Here's how the part is built. I have some questions about the finished solid (model axes, mm). A direction names the side the tool comes from. Give positions to 0.01 mm unless a question says otherwise; leave off trailing zeros. Write each loop counter-clockwise with the first axis right and the second up, starting at its lowest first coordinate (ties: lowest second). Pieces come first, ordered by that corner, then holes. Notation, with made-up numbers: (-4, 58.5) - (35, 58.5) arc R34 cw to (35, 94.5) - close; hole circle Ø4 at (-26, 36.25). An arc over 180 degrees is marked (long way). One line per item, written item: value. Start each with the question number.
1) Imagine slicing it at A-A on z = -28.5. Write out the boundary of the cut face in (x, y).
2) Please list where these lines run through material, in increasing order: L1, parallel to Y at x = 14, z = -36; L2, parallel to Z at x = 18.5, y = 331. Write a range as [from, to].
3) We'd pull the mould along Y, two halves only. Please class faces 1 (the flat face through (0, 572, -44)), 2 (the flat face through (44, 290, -22)), 3 (the flat face through (44, 1160, -46)), 4 (the flat face through (44, 780, -22)): +Y half, -Y half, draft (parallel to the pull), parting line (faces both ways), or undercut.
4) Imagine slicing it at B-B on x = 46. Write out the boundary of the cut face in (y, z), plus the area to 3 significant figures.
5) On a 3-axis mill with a long thin cutter (end or side, diameter ignored), from which of +Z, -Z, +X, -X, +Y, -Y can I reach the whole of each face in a straight line? I mean faces 5 (the flat face through (44, 577, 0)), 6 (the flat face through (44, 380, -22)). Say none if no direction works.
from build123d import *

# Parameters (mm, degrees)
SKETCH1_W           = 90
SKETCH1_H           = 90
BOSS_EXTRUDE1_DEPTH = 1160
SKETCH3_W           = 90
SKETCH3_H           = 90
CUT_EXTRUDE1_DEPTH  = 45
SKETCH4_W           = 90
SKETCH4_H           = 90
CUT_EXTRUDE2_DEPTH  = 45


with BuildPart() as part:
    # Sketch1 → Boss-Extrude1 (new body)
    with BuildSketch(Plane(origin=(0, 0, 0), x_dir=(1, 0, 0), z_dir=(0, 1, 0))):
        with Locations((45, 45)):
            Rectangle(SKETCH1_W, SKETCH1_H)
    extrude(amount=BOSS_EXTRUDE1_DEPTH)

    # Sketch3 → Cut-Extrude1 (cut)
    with BuildSketch(Plane.XY):
        with Locations((45, 825)):
            Rectangle(SKETCH3_W, SKETCH3_H)
    extrude(amount=-CUT_EXTRUDE1_DEPTH, mode=Mode.SUBTRACT)

    # Sketch4 → Cut-Extrude2 (cut)
    with BuildSketch(Plane.XY):
        with Locations((45, 335)):
            Rectangle(SKETCH4_W, SKETCH4_H)
    extrude(amount=-CUT_EXTRUDE2_DEPTH, mode=Mode.SUBTRACT)


solid = part.part
Numbers:
1. outline: (0, 0) - (90, 0) - (90, 290) - (0, 290) - close; (0, 380) - (90, 380) - (90, 780) - (0, 780) - close; (0, 870) - (90, 870) - (90, 1160) - (0, 1160) - close
2. L1: [0, 290], [380, 780], [870, 1160]
2. L2: [-90, -45]
3. face 1: draft
3. face 2: undercut
3. face 3: +Y half
3. face 4: undercut
4. outline: (0, -90) - (1160, -90) - (1160, 0) - (870, 0) - (870, -45) - (780, -45) - (780, 0) - (380, 0) - (380, -45) - (290, -45) - (290, 0) - (0, 0) - close
4. area: 96,300 mm^2
5. face 5: +Z, +X, -X, +Y, -Y
5. face 6: +Z, +X, -X
